from build123d import *

# Parameters (mm, degrees)
SKETCH1_W           = 65
SKETCH1_H           = 64
SKETCH1_R           = 1.15
BOSS_EXTRUDE1_DEPTH = 3
BOSS_EXTRUDE2_DEPTH = 3.8


with BuildPart() as part:
    # Sketch1 → Boss-Extrude1 (new body)
    with BuildSketch(Plane(origin=(0, 0, 0), x_dir=(1, 0, 0), z_dir=(0, 1, 0))):
        with Locations((-2.334951456, -14.330097087)):
            Rectangle(SKETCH1_W, SKETCH1_H)
        with Locations(Location((-32.234951456, 15.019902913, 0), (0, 0, 270))):
            Circle(SKETCH1_R, mode=Mode.SUBTRACT)
        with Locations(Location((27.565048544, 15.019902913, 0), (0, 0, 270))):
            Circle(SKETCH1_R, mode=Mode.SUBTRACT)
        with Locations(Location((-32.234951456, -43.680097087, 0), (0, 0, 270))):
            Circle(SKETCH1_R, mode=Mode.SUBTRACT)
        with Locations(Location((27.565048544, -43.680097087, 0), (0, 0, 270))):
            Circle(SKETCH1_R, mode=Mode.SUBTRACT)
    extrude(amount=BOSS_EXTRUDE1_DEPTH)

    # Sketch2 → Boss-Extrude2 (add)
    with BuildSketch(Plane(origin=(0, 3, 0), x_dir=(1, 0, 0), z_dir=(0, 1, 0))):
        with BuildLine():
            Line((-30.334951456, 14.169902913), (25.665048544, 14.169902913))
            ThreePointArc((25.665048544, 14.169902913), (27.079262106, 13.584116475), (27.665048544, 12.169902913))
            Line((27.665048544, 12.169902913), (27.665048544, -40.830097087))
            ThreePointArc((27.665048544, -40.830097087), (27.079262106, -42.24431065), (25.665048544, -42.830097087))
            Line((25.665048544, -42.830097087), (-30.334951456, -42.830097087))
            ThreePointArc((-30.334951456, -42.830097087), (-31.749165019, -42.24431065), (-32.334951456, -40.830097087))
            Line((-32.334951456, -40.830097087), (-32.334951456, 12.169902913))
            ThreePointArc((-32.334951456, 12.169902913), (-31.749165019, 13.584116475), (-30.334951456, 14.169902913))
        make_face()
    extrude(amount=BOSS_EXTRUDE2_DEPTH)


solid = part.part
Model file for the job. Use its own axes, mm. A direction names the side the tool comes from. Give positions to 0.01 mm unless a question says otherwise; leave off trailing zeros. Order: outer loops, then holes, each group sorted by start corner. A loop starts at its lowest first (then second) coordinate and runs counter-clockwise, first axis right, second up. Notation, with made-up numbers: M 27.5,2.25 L 52.5,2.25 A15 cw 52.5,23.25 Z; hole C -12.75,56.25 d5. An arc over 180 degrees is marked long. Put each result on its own line as item: value. Start each with the question number.
(1) Tool access for faces 1 (the face through (-32.335, 5, 15)), 2 (the face through (-3, 5, -14.17)), 3 (the face through (-2, 5, 42.83)), 4 (the face through (-31.765, 4.873, -13.568)): list every direction of +Z, -Z, +X, -X, +Y, -Y with a clear straight run to the whole face (end or side of a thin tool).
(2) Pull direction X, two halves, no side cores. Call faces 5 (the face through (-31.734, 4.873, 42.26)), 6 (the face through (27.665, 5, 14)), 7 (the face through (-32.18, 1.48, 42.53)): released by +X, released by -X, zero draft, split by the parting line, or undercut.
(3) Band-saw the part on B-B on y = 4. Give the cut face in (x, z), then the cut area to 3 significant figures.
(4) Band-saw the part on A-A on x = -11. Give the cut face in (y, z), then the cut area to 3 significant figures.
(5) Pin check, flat tips, straight feed: pin 1 Ø1.1 at (y, z) = (5, 3) entering from -X; pin 2 Ø1.9 at (y, z) = (5, 25) entering from +X; pin 3 Ø1.1 at (x, y) = (-2, 5.5) entering from -Z. Stop position of each tip, or through.
(6) Drill centre lines: L1, parallel to Z at x = 8, y = 4.5; L2, parallel to X at y = 4, z = 24; L3, parallel to X at y = 4, z = -13. Where is each one in solid material? Low to high. Write a range as [from, to].
Results below:
1. face 1: +Z, -Z, -X, +Y
1. face 2: -Z, +X, -X, +Y
1. face 3: +Z, +X, -X, +Y
1. face 4: -Z, -X, +Y
2. face 5: released by -X
2. face 6: released by +X
2. face 7: undercut
3. outline: M -32.33,-12.17 A2 ccw -30.33,-14.17 L 25.67,-14.17 A2 ccw 27.67,-12.17 L 27.67,40.83 A2 ccw 25.67,42.83 L -30.33,42.83 A2 ccw -32.33,40.83 Z
3. area: 3,420 mm2
4. outline: M 0,-17.67 L 3,-17.67 L 3,-14.17 L 6.8,-14.17 L 6.8,42.83 L 3,42.83 L 3,46.33 L 0,46.33 Z
4. area: 409 mm2
5. pin 1: stops at x = -32.33
5. pin 2: stops at x = 27.67
5. pin 3: stops at z = -14.17
6. L1: z = [-14.17, 42.83]
6. L2: x = [-32.33, 27.67]
6. L3: x = [-32.15, 27.48]
